from build123d import *

# Parameters (mm, degrees)
SKETCH1_W                = 15
SKETCH1_H                = 15
BOSS_EXTRUDE1_DEPTH      = 35
SKETCH3_W                = 7
SKETCH3_H                = 15
CUT_EXTRUDE1_DEPTH       = 12
SKETCH4_R                = 2
CUT_EXTRUDE2_DEPTH       = 15
SKETCH5_W                = 4
SKETCH5_H                = 15
CUT_EXTRUDE3_DEPTH       = 15
BOSS_EXTRUDE2_DEPTH      = 7.5
BOSS_EXTRUDE2_DEPTH_BACK = 7.5
SKETCH6_R                = 2
FILLET1_R                = 7.5
CUT_EXTRUDE6_DEPTH       = 3.5
CUT_EXTRUDE6_DEPTH_BACK  = 3.5
FILLET2_R                = 2
CUT_EXTRUDE7_DEPTH       = 7.5
CUT_EXTRUDE7_DEPTH_BACK  = 7.5
FILLET3_SIZE             = 4
FILLET3_SIZE_2           = 2
CUT_EXTRUDE8_DEPTH       = 1
CUT_EXTRUDE8_DEPTH_BACK  = 1


# Some blends are built 0.0001 mm under size
with BuildPart() as part:
    # Sketch1 → Boss-Extrude1 (new body)
    with BuildSketch(Plane.XY):
        Rectangle(SKETCH1_W, SKETCH1_H)
    extrude(amount=BOSS_EXTRUDE1_DEPTH)

    # Sketch3 → Cut-Extrude1 (cut)
    with BuildSketch(Plane.XY.offset(35)):
        Rectangle(SKETCH3_W, SKETCH3_H)
    extrude(amount=-CUT_EXTRUDE1_DEPTH, mode=Mode.SUBTRACT)

    # Sketch4 → Cut-Extrude2 (cut)
    with BuildSketch(Plane(origin=(7.5, 0, 0), x_dir=(0, 0, -1), z_dir=(1, 0, 0))):
        with Locations(Location((-27.5, 0, 0), (0, 0, 90))):
            Circle(SKETCH4_R)
    extrude(amount=-CUT_EXTRUDE2_DEPTH, mode=Mode.SUBTRACT)

    # Sketch5 → Cut-Extrude3 (cut)
    with BuildSketch(Plane(origin=(0, 0, 0), x_dir=(-1, 0, 0), z_dir=(0, 0, -1))):
        with Locations((-5.5, 0)):
            Rectangle(SKETCH5_W, SKETCH5_H)
        with Locations((5.5, 0)):
            Rectangle(SKETCH5_W, SKETCH5_H)
    extrude(amount=-CUT_EXTRUDE3_DEPTH, mode=Mode.SUBTRACT)

    # Sketch6 → Boss-Extrude2 (add, two sides: drawn at the far end of the back side and taken through both)
    with BuildSketch(Plane(origin=(0, 0, 0), x_dir=(0, 0, -1), z_dir=(1, 0, 0)).offset(-BOSS_EXTRUDE2_DEPTH_BACK)):
        with Locations((-7.5, 0)):
            Circle(SKETCH6_R)
    extrude(amount=BOSS_EXTRUDE2_DEPTH + BOSS_EXTRUDE2_DEPTH_BACK)

    # Fillet1
    fillet1_edges = [part.edges().sort_by_distance(p)[0] for p in [
        (5.5, -7.5, 35),
        (-5.5, -7.5, 35),
        (-5.5, 7.5, 35),
        (5.5, 7.5, 35),
    ]]
    fillet(fillet1_edges, radius=FILLET1_R - 0.0001)  # a hair under: the kernel refuses the full size

    # Sketch7 → Cut-Extrude6 (cut, two sides: drawn at the far end of the back side and taken through both)
    with BuildSketch(Plane(origin=(0, 0, 0), x_dir=(0, 0, -1), z_dir=(1, 0, 0)).offset(-CUT_EXTRUDE6_DEPTH_BACK)):
        Polygon((-23, 7.5), (-23, 4.5), (-20, 7.5), align=None)
    extrude(amount=CUT_EXTRUDE6_DEPTH + CUT_EXTRUDE6_DEPTH_BACK, mode=Mode.SUBTRACT)

    # Fillet2
    fillet2_edges = [part.edges().sort_by_distance(p)[0] for p in [
        (7.5, -7.5, 21.25005),
        (7.5, 7.5, 21.25005),
        (7.5, 5.303330148, 32.803330148),
        (7.5, -5.303330148, 32.803330148),
        (-7.5, -7.5, 21.25005),
        (-7.5, 7.5, 21.25005),
        (-7.5, 5.303330148, 32.803330148),
        (-7.5, -5.303330148, 32.803330148),
    ]]
    fillet(fillet2_edges, radius=FILLET2_R)

    # Sketch8 → Cut-Extrude7 (cut, two sides: drawn at the far end of the back side and taken through both)
    with BuildSketch(Plane(origin=(0, 0, 0), x_dir=(0, 0, -1), z_dir=(1, 0, 0)).offset(-CUT_EXTRUDE7_DEPTH_BACK)):
        with BuildLine():
            Line((-15, 7.5), (-12, 4.5))
            Line((-12, 4.5), (-7.5, 4.5))
            ThreePointArc((-7.5, 4.5), (-4.318019485, 3.181980515), (-3, 0))
            Line((-3, 0), (-3, -7.5))
            Line((-3, -7.5), (0, -7.5))
            Line((0, -7.5), (0, 7.5))
            Line((0, 7.5), (-15, 7.5))
        make_face()
    extrude(amount=CUT_EXTRUDE7_DEPTH + CUT_EXTRUDE7_DEPTH_BACK, mode=Mode.SUBTRACT)

    # Fillet3
    # an asymmetric fillet: 4, 2 mm, written as the material it takes off along each edge
    with BuildSketch(Plane(origin=(-13.5, -7.5, 3), x_dir=(0, 0, 1), z_dir=(1, 0, 0))) as fillet3_piece_1:
        with BuildLine():
            Bezier((FILLET3_SIZE, 0), (0, 0), (0, -FILLET3_SIZE_2), weights=[1, 0.707106781, 1])
            Line((0, -FILLET3_SIZE_2), (0, 0))
            Line((0, 0), (FILLET3_SIZE, 0))
        make_face()
    extrude(amount=27, mode=Mode.SUBTRACT)

    # Sketch9 → Cut-Extrude8 (cut, two sides: drawn at the far end of the back side and taken through both)
    with BuildSketch(Plane(origin=(0, 0, 0), x_dir=(0, 0, -1), z_dir=(1, 0, 0)).offset(-CUT_EXTRUDE8_DEPTH_BACK)):
        with BuildLine():
            Line((-8, -0.5), (-8, 9.147620524))
            ThreePointArc((-8, 9.147620524), (-1.178102105, 6.321897895), (1.647620524, -0.5))
            Line((1.647620524, -0.5), (-8, -0.5))
        make_face()
    extrude(amount=CUT_EXTRUDE8_DEPTH + CUT_EXTRUDE8_DEPTH_BACK, mode=Mode.SUBTRACT)


solid = part.part
The listing builds one solid part. Answer for the finished solid, in the listing's coordinates (mm). A direction names the side the tool comes from. Round coordinates to 2 decimals unless told otherwise and drop trailing zeros. Order: outer loops, then holes, each group sorted by start corner. A loop starts at its lowest first (then second) coordinate and runs counter-clockwise, first axis right, second up. Notation, with made-up numbers: M -36,27.5 L -22,27.5 A27 cw -22,57.5 Z; hole C 25,59 d5. An arc over 180 degrees is marked long. Answer in a Markdown table with one row per item. Add a question column.
1) Flat-ended cylindrical pins translate along their axes: pin 1 Ø0.6 at (x, z) = (-0.5, 5) entering from +Y; pin 2 Ø6 at (x, y) = (3, 4) entering from -Z; pin 3 Ø1.2 at (x, y) = (-6, 0) entering from -Z; pin 4 Ø3 at (y, z) = (0, 27.5) entering from -X. Find the tip coordinate at first contact, or state that the pin passes through.
2) The part is cut by section A-A on x = 4. Count the separate pieces of the cut face and the enclosed holes in it, plus the area to 3 significant figures.
3) Which of the six approach directions +Z, -Z, +X, -X, +Y, -Y give full straight-line access (tool end or side, diameter ignored) to faces 1 (the face through (6, 0, 15)), 2 (the face through (-5, 0, 15)), 3 (the face through (0, 4.5, 10)), 4 (the face through (0, 2, 8))?
4) Determine the mould class of faces 5 (the face through (3.5, -2, 9)), 6 (the face through (-3.5, 2, 29)), 7 (the face through (4.514, -5.361, 32.745)), 8 (the face through (-6.9, -6.93, 21.34)) for opening direction X: pulls with the +X half, pulls with the -X half, needs draft (parallel to the pull), parting line crosses it, or undercut.
5) Consider line 1 along Z through (x, y) = (-4.6, 0); line 2 along Z through (x, y) = (6.35, 0); line 3 along X through (y, z) = (2.5, 27.5). Determine where each line is inside the solid, lowest interval first. Write a range as from..to.
6) The part is cut by section B-B on z = 17. Determine the outline of the cut face in (x, y), plus the area to 3 significant figures.
Findings below:
| question | item | result |
|---|---|---|
| 1 | pin 1 | stops at y = -0.5 |
| 1 | pin 2 | stops at z = 3.11 |
| 1 | pin 3 | stops at z = 5.5 |
| 1 | pin 4 | passes through |
| 2 | separate pieces | 2 |
| 2 | enclosed holes | 1 |
| 2 | area | 276 mm² |
| 3 | face 1 | +X, +Y, -Y |
| 3 | face 2 | -X, +Y, -Y |
| 3 | face 3 | -Z, +X, -X, +Y |
| 3 | face 4 | -Z, +Y |
| 4 | face 5 | pulls with the +X half |
| 4 | face 6 | undercut |
| 4 | face 7 | needs draft |
| 4 | face 8 | pulls with the -X half |
| 5 | line 1 | z = 5.5..9.5, 15..25.5, 29.5..35 |
| 5 | line 2 | z = 5.5..9.5, 15..25.5, 29.5..34.81 |
| 5 | line 3 | x = -7.5..-3.5, 3.5..7.5 |
| 6 | outline | M -7.5,-5.5 A2 ccw -5.5,-7.5 L 5.5,-7.5 A2 ccw 7.5,-5.5 L 7.5,5.5 A2 ccw 5.5,7.5 L -5.5,7.5 A2 ccw -7.5,5.5 Z |
| 6 | area | 222 mm² |
